Here's how the part is built. I have some questions about the finished solid (model axes, mm). Coordinates: 2 decimals unless noted, no trailing zeros. Order: outer loops, then holes, each group sorted by start corner. A loop starts at its lowest first (then second) coordinate and runs counter-clockwise, first axis right, second up. Notation, with made-up numbers: (-16.5, 48) - (9.5, 48) arc R25 cw to (9.5, 79) - close; hole circle Ø3 at (87.25, 54). An arc over 180 degrees is marked (long way). Use CSV: the item, a comma, the result in double quotes. Start each with the question number.
from build123d import *

# Parameters (mm, degrees)
SKETCH5_W           = 58.25
SKETCH5_H           = 91.35
SKETCH5_R           = 1.15
SKETCH5_R_2         = 1.6
SKETCH5_W_2         = 38.25
SKETCH5_H_2         = 23.65
BOSS_EXTRUDE1_DEPTH = 2.5
SKETCH8_W           = 4.5
SKETCH8_H           = 10
SKETCH8_W_2         = 3
SKETCH8_H_2         = 3
CUT_EXTRUDE1_DEPTH  = 1
FILLET1_R           = 2
FILLET2_R           = 5
SKETCH9_W           = 6.8
SKETCH9_H           = 12.1
CUT_EXTRUDE2_DEPTH  = 55.228417366
SKETCH10_W          = 7.2
SKETCH10_H          = 5.49
CUT_EXTRUDE3_DEPTH  = 1
FILLET3_R           = 0.8
CHAMFER3_SIZE       = 1


with BuildPart() as part:
    # Sketch5 → Boss-Extrude1 (new body)
    with BuildSketch(Plane(origin=(0, 0, 0), x_dir=(1, 0, 0), z_dir=(0, 1, 0))):
        Rectangle(SKETCH5_W, SKETCH5_H)
        with Locations(Location((-17.23, 5.255, 0), (0, 0, 270))):
            Circle(SKETCH5_R, mode=Mode.SUBTRACT)
        with Locations(Location((-24.125, 40.675, 0), (0, 0, 270))):
            Circle(SKETCH5_R_2, mode=Mode.SUBTRACT)
        with Locations(Location((-24.125, -40.675, 0), (0, 0, 270))):
            Circle(SKETCH5_R_2, mode=Mode.SUBTRACT)
        with Locations(Location((24.125, -34.325, 0), (0, 0, 270))):
            Circle(SKETCH5_R_2, mode=Mode.SUBTRACT)
        with Locations(Location((24.125, 40.675, 0), (0, 0, 270))):
            Circle(SKETCH5_R_2, mode=Mode.SUBTRACT)
        with Locations(Location((16.23, 5.255, 0), (0, 0, 270))):
            Circle(SKETCH5_R, mode=Mode.SUBTRACT)
        with Locations(Location((16.23, -26.805, 0), (0, 0, 270))):
            Circle(SKETCH5_R, mode=Mode.SUBTRACT)
        with Locations(Location((-17.23, -26.805, 0), (0, 0, 270))):
            Circle(SKETCH5_R, mode=Mode.SUBTRACT)
        Polygon((-19.125, 2.025), (19.125, 2.025), (19.125, -22.805), (12.23, -22.805), (12.23, -30.805), (19.125, -30.805), (19.125, -35.675), (-19.125, -35.675), (-19.125, -31.805), (-12.23, -31.805), (-12.23, -21.805), (-19.125, -21.805), align=None, mode=Mode.SUBTRACT)
        with Locations((0, 23.85)):
            Rectangle(SKETCH5_W_2, SKETCH5_H_2, mode=Mode.SUBTRACT)
    extrude(amount=BOSS_EXTRUDE1_DEPTH)

    # Sketch8 → Cut-Extrude1 (cut)
    with BuildSketch(Plane(origin=(0, 2.5, 0), x_dir=(1, 0, 0), z_dir=(0, 1, 0))):
        with Locations((20.65, -21.675)):
            Rectangle(SKETCH8_W, SKETCH8_H)
        with Locations((5, 7.075)):
            Rectangle(SKETCH8_W_2, SKETCH8_H_2)
    extrude(amount=-CUT_EXTRUDE1_DEPTH, mode=Mode.SUBTRACT)

    # Fillet1
    # the kernel refuses this fillet: 2 mm, written as the material it adds along each edge
    with BuildSketch(Plane(origin=(19.125, 0, -12.025), x_dir=(0, 0, -1), z_dir=(0, 1, 0)), Plane(origin=(19.125, 0, -35.675), x_dir=(-1, 0, 0), z_dir=(0, 1, 0)), Plane(origin=(-19.125, 0, -35.675), x_dir=(0, 0, 1), z_dir=(0, 1, 0)), Plane(origin=(19.125, 0, -2.025), x_dir=(-1, 0, 0), z_dir=(0, 1, 0)), Plane(origin=(-19.125, 0, 21.805), x_dir=(1, 0, 0), z_dir=(0, 1, 0)), Plane(origin=(19.125, 0, 30.805), x_dir=(-1, 0, 0), z_dir=(0, 1, 0)), Plane(origin=(-19.125, 0, 31.805), x_dir=(0, 0, 1), z_dir=(0, 1, 0)), Plane(origin=(-19.125, 0, 35.675), x_dir=(1, 0, 0), z_dir=(0, 1, 0))) as fillet1_piece_1:
        with BuildLine():
            CenterArc((FILLET1_R, FILLET1_R), FILLET1_R, 180, 90)
            Line((0, FILLET1_R), (0, 0))
            Line((0, 0), (FILLET1_R, 0))
        make_face()
    extrude(amount=2.5)
    with BuildSketch(Plane(origin=(-19.125, 0, -12.025), x_dir=(0, 0, -1), z_dir=(0, 1, 0)), Plane(origin=(-19.125, 0, -2.025), x_dir=(1, 0, 0), z_dir=(0, 1, 0))) as fillet1_piece_2:
        with BuildLine():
            CenterArc((FILLET1_R, -FILLET1_R), FILLET1_R, 90, 90)
            Line((0, -FILLET1_R), (0, 0))
            Line((0, 0), (FILLET1_R, 0))
        make_face()
    extrude(amount=2.5)
    with BuildSketch(Plane(origin=(19.125, 0, 22.805), x_dir=(0, 0, -1), z_dir=(0, 1, 0))) as fillet1_piece_3_section:
        with BuildLine():
            CenterArc((FILLET1_R, FILLET1_R), FILLET1_R, 180, 90)
            Line((0, FILLET1_R), (0, 0))
            Line((0, 0), (FILLET1_R, 0))
        make_face()
    fillet1_piece_3 = extrude(amount=1.5, mode=Mode.PRIVATE)
    fillet1_piece_3 = split(fillet1_piece_3, bisect_by=Plane(origin=(18.4, 0.75, 22.246257115), z_dir=(1, 0, 0)), keep=Keep.TOP, mode=Mode.PRIVATE)
    add(fillet1_piece_3)
    with BuildSketch(Plane(origin=(19.125, 0, 22.805), x_dir=(0, 0, -1), z_dir=(0, 1, 0))) as fillet1_piece_4_section:
        with BuildLine():
            CenterArc((FILLET1_R, FILLET1_R), FILLET1_R, 180, 90)
            Line((0, FILLET1_R), (0, 0))
            Line((0, 0), (FILLET1_R, 0))
        make_face()
    fillet1_piece_4 = extrude(amount=1.5, mode=Mode.PRIVATE)
    fillet1_piece_4 = split(fillet1_piece_4, bisect_by=Plane(origin=(18.4, 0.75, 22.70384679), z_dir=(-1, 0, 0)), keep=Keep.TOP, mode=Mode.PRIVATE)
    add(fillet1_piece_4)
    with BuildSketch(Plane(origin=(19.125, 0, 22.805), x_dir=(0, 0, -1), z_dir=(0, 1, 0))) as fillet1_piece_5_section:
        with BuildLine():
            CenterArc((FILLET1_R, FILLET1_R), FILLET1_R, 180, 90)
            Line((0, FILLET1_R), (0, 0))
            Line((0, 0), (FILLET1_R, 0))
        make_face()
    fillet1_piece_5 = extrude(amount=6.5, mode=Mode.PRIVATE)
    fillet1_piece_5 = split(fillet1_piece_5, bisect_by=Plane(origin=(18.018520093, 2.5, 22.70384679), z_dir=(0, -1, 0)), keep=Keep.TOP, mode=Mode.PRIVATE)
    fillet1_piece_5 = split(fillet1_piece_5, bisect_by=Plane(origin=(18.018520093, 1.5, 22.70384679), z_dir=(0, 1, 0)), keep=Keep.TOP, mode=Mode.PRIVATE)
    fillet1_piece_5 = split(fillet1_piece_5, bisect_by=Plane(origin=(18.4, 2, 22.70384679), z_dir=(-1, 0, 0)), keep=Keep.TOP, mode=Mode.PRIVATE)
    add(fillet1_piece_5)
    # the kernel refuses this fillet: 2 mm, written as the material it takes off along each edge
    with BuildSketch(Plane(origin=(12.23, -5, 30.805), x_dir=(1, 0, 0), z_dir=(0, 1, 0)), Plane(origin=(12.23, -5, 22.805), x_dir=(0, 0, 1), z_dir=(0, 1, 0)), Plane(origin=(-12.23, -5, 31.805), x_dir=(0, 0, -1), z_dir=(0, 1, 0)), Plane(origin=(-12.23, -5, 21.805), x_dir=(-1, 0, 0), z_dir=(0, 1, 0))) as fillet1_2_piece_1:
        with BuildLine():
            CenterArc((FILLET1_R, FILLET1_R), FILLET1_R, 180, 90)
            Line((0, FILLET1_R), (0, 0))
            Line((0, 0), (FILLET1_R, 0))
        make_face()
    extrude(amount=12.5, mode=Mode.SUBTRACT)

    # Fillet2
    fillet2_edges = [part.edges().sort_by_distance(p)[0] for p in [
        (29.125, 1.25, -45.675),
        (29.125, 1.25, 45.675),
        (-29.125, 1.25, 45.675),
        (-29.125, 1.25, -45.675),
    ]]
    fillet(fillet2_edges, radius=FILLET2_R)

    # Sketch9 → Cut-Extrude2 (cut, through all)
    with BuildSketch(Plane.XZ):
        with Locations((-17.7, 6.125)):
            Rectangle(SKETCH9_W, SKETCH9_H)
    extrude(amount=-CUT_EXTRUDE2_DEPTH, mode=Mode.SUBTRACT)

    # Sketch10 → Cut-Extrude3 (cut)
    with BuildSketch(Plane(origin=(0, 0, 0), x_dir=(1, 0, 0), z_dir=(0, 1, 0))):
        with Locations((0.325, 6.42)):
            Rectangle(SKETCH10_W, SKETCH10_H)
    extrude(amount=CUT_EXTRUDE3_DEPTH, mode=Mode.SUBTRACT)

    # Fillet3
    fillet3_edges = [part.edges().sort_by_distance(p)[0] for p in [
        (-19.125, 1.25, 12.175),
        (-21.1, 1.25, 12.175),
        (-19.125, 1.25, 0.075),
        (-21.1, 1.25, 0.075),
        (3.925, 0.5, -3.675),
        (3.925, 0.5, -9.165),
        (-3.275, 0.5, -9.165),
        (-3.275, 0.5, -3.675),
        (18.4, 2, 26.675),
    ]]
    fillet(fillet3_edges, radius=FILLET3_R)

    # Chamfer3
    chamfer3_edges = [part.edges().sort_by_distance(p)[0] for p in [
        (29.125, 2.5, 0),
        (0, 2.5, 45.675),
        (0, 2.5, -45.675),
        (-29.125, 2.5, 0),
        (27.660533906, 2.5, -44.210533906),
        (-27.660533906, 2.5, -44.210533906),
        (-27.660533906, 2.5, 44.210533906),
        (27.660533906, 2.5, 44.210533906),
    ]]
    chamfer(chamfer3_edges, length=CHAMFER3_SIZE)


solid = part.part
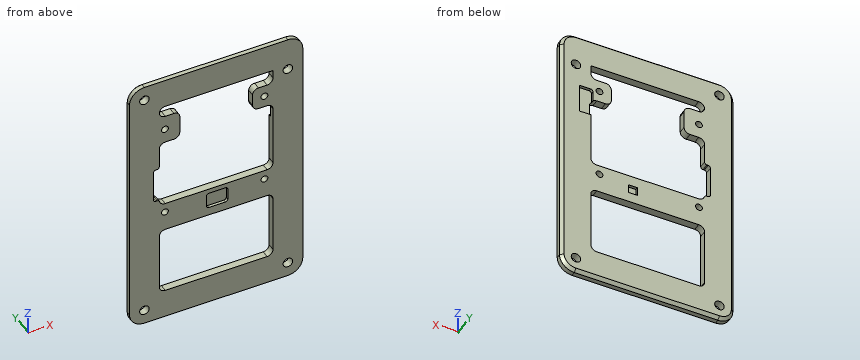
Item 1: Please list where these lines run through material, in increasing order: line 1 along Z through (x, y) = (-11, 1) (3 decimals); line 2 along Z through (x, y) = (-13.5, 0.55) (3 decimals); line 3 along X through (y, z) = (0.6, 7) (3 decimals). Write a range as from..to.
Item 2: Suppose I cut it at B-B on z = 14. Write out the boundary of the cut face in (x, y) (3 decimals), then the cut area to 3 significant figures.
Item 3: For pin 1 Ø1.6 at (x, z) = (1, -5.5) entering from -Y; pin 2 Ø1.8 at (x, z) = (-17.23, 26.805) entering from +Y, each with a flat end and sliding along its axis, tell me the tip position at first contact or that it passes through.
Item 4: Suppose I cut it at A-A on x = 16.23. Write out the boundary of the cut face in (y, z) (3 decimals), then the cut area to 3 significant figures.
Here are the results:
1,line 1,"-45.675..-35.675, -12.025..-2.025, 35.675..45.675"
1,line 2,"-45.675..-35.675, -12.025..-2.025, 21.943..31.667, 35.675..45.675"
1,line 3,"-29.125..-21.1, 19.125..29.125"
2,outline,"(-29.125, 0) - (-19.125, 0) - (-19.125, 2.5) - (-28.125, 2.5) - (-29.125, 1.5) - close; (19.125, 0) - (29.125, 0) - (29.125, 1.5) - (28.125, 2.5) - (19.125, 2.5) - close"
2,area,"49.0 mm^2"
3,pin 1,"y = 1"
3,pin 2,"through"
4,outline,"(0, -45.675) - (1.5, -45.675) - (2.5, -44.675) - (2.5, -35.675) - (0, -35.675) - close; (0, -12.025) - (2.5, -12.025) - (2.5, -6.405) - (0, -6.405) - close; (0, -4.105) - (2.5, -4.105) - (2.5, -2.025) - (0, -2.025) - close; (0, 22.805) - (2.5, 22.805) - (2.5, 25.655) - (0, 25.655) - close; (0, 27.955) - (2.5, 27.955) - (2.5, 30.805) - (0, 30.805) - close; (0, 35.675) - (2.5, 35.675) - (2.5, 44.675) - (1.5, 45.675) - (0, 45.675) - close"
4,area,"82.5 mm^2"
